Verification items for this drawing (mm, ordinates from the low corner). Give positions to 0.01 mm unless a question says otherwise; leave off trailing zeros. Loops run counter-clockwise (first coordinate to the right, second up) from the corner with the lowest first, then second, coordinate; pieces in that order, holes last. Notation, with made-up numbers: (21, -19.75) -> (31, -19.75) arc R22 ccw to (31, -7.75) -> close; hole circle Ø8 at (-26, 56). An arc over 180 degrees is marked (long way). Answer as CSV lines item,"result". Start each with the question number.
(1) Section check A-A on x = 5. Enter the section's corners in (y, z), plus the area to 3 significant figures.
(2) Material ranges on line 1 (Z direction, x = 3.5, y = 3.25); line 2 (Y direction, x = 2.75, z = 41.8); line 3 (Z direction, x = 3.25, y = 3.5), recorded low to high. Write a range as from..to.
(3) Section check C-C on z = 31. Enter the section's corners in (x, y), plus the area to 3 significant figures.
(4) Section check B-B on y = 5. Enter the section's corners in (x, z).
(5) Section check D-D on z = 41.8. Enter the section's corners in (x, y), plus the area to 3 significant figures.
(6) Release check for a two-part mould opening along X. For the marked faces 1 and 2 record: pulls with the +X half, pulls with the -X half, needs draft (parallel to the pull), parting line crosses it, or undercut.
(7) Gauge pin test, flat ends, axial feed: pin 1 Ø1 at (x, z) = (6.5, 5) entering from -Y; pin 2 Ø3 at (x, z) = (7.5, 35) entering from +Y. Record the tip position at first contact, or that the pin passes through.
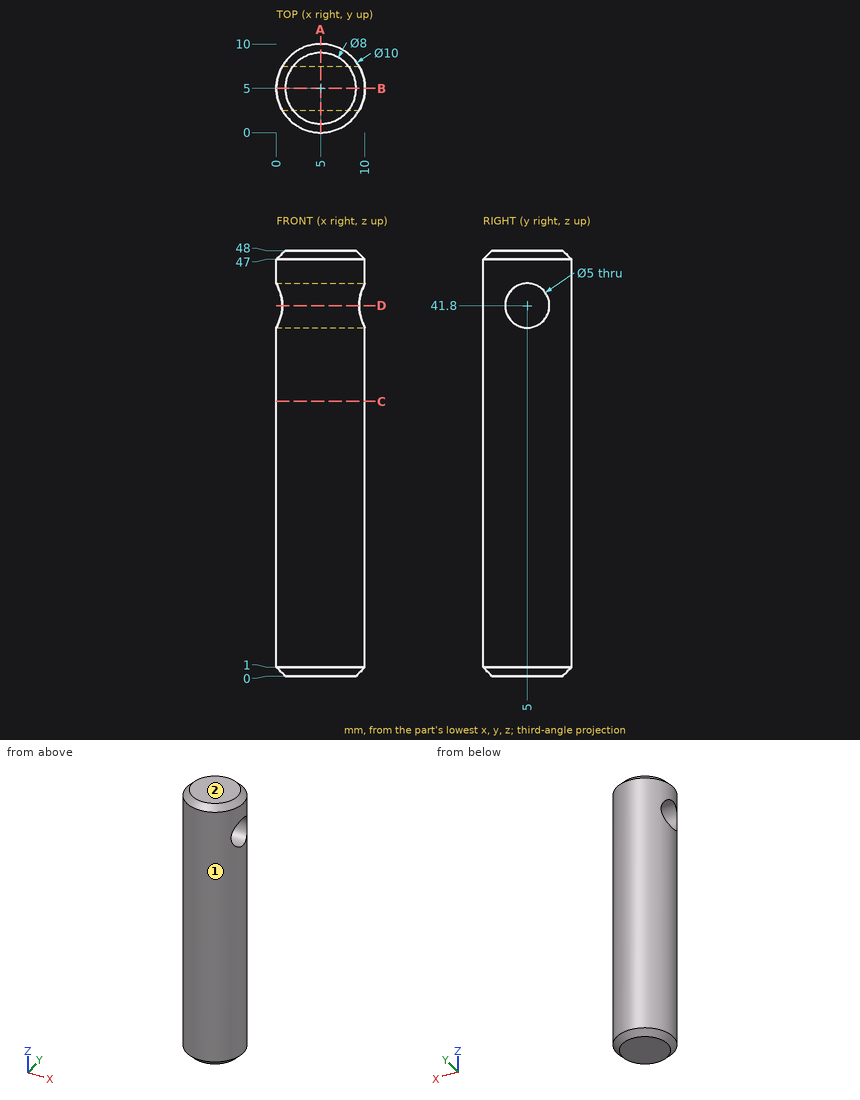
Working result:
1,outline,"(0, 1) -> (1, 0) -> (9, 0) -> (10, 1) -> (10, 47) -> (9, 48) -> (1, 48) -> (0, 47) -> close; hole circle Ø5 at (5, 41.8)"
1,area,"458 mm^2"
2,line 1,"z = 0..40.01, 43.59..48"
2,line 2,"y = 0.53..2.5, 7.5..9.47"
2,line 3,"z = 0..39.8, 43.8..48"
3,outline,"circle Ø10 at (5, 5)"
3,area,"78.5 mm^2"
4,outline,"(0, 1) -> (1, 0) -> (9, 0) -> (10, 1) -> (10, 39.3) -> (0, 39.3) -> close; (0, 44.3) -> (10, 44.3) -> (10, 47) -> (9, 48) -> (1, 48) -> (0, 47) -> close"
5,outline,"(0.67, 2.5) arc R5 ccw to (9.33, 2.5) -> close; (0.67, 7.5) -> (9.33, 7.5) arc R5 ccw to start"
5,area,"30.7 mm^2"
6,face 1,"parting line crosses it"
6,face 2,"needs draft"
7,pin 1,"stops at y = 0.1"
7,pin 2,"stops at y = 9.9"
